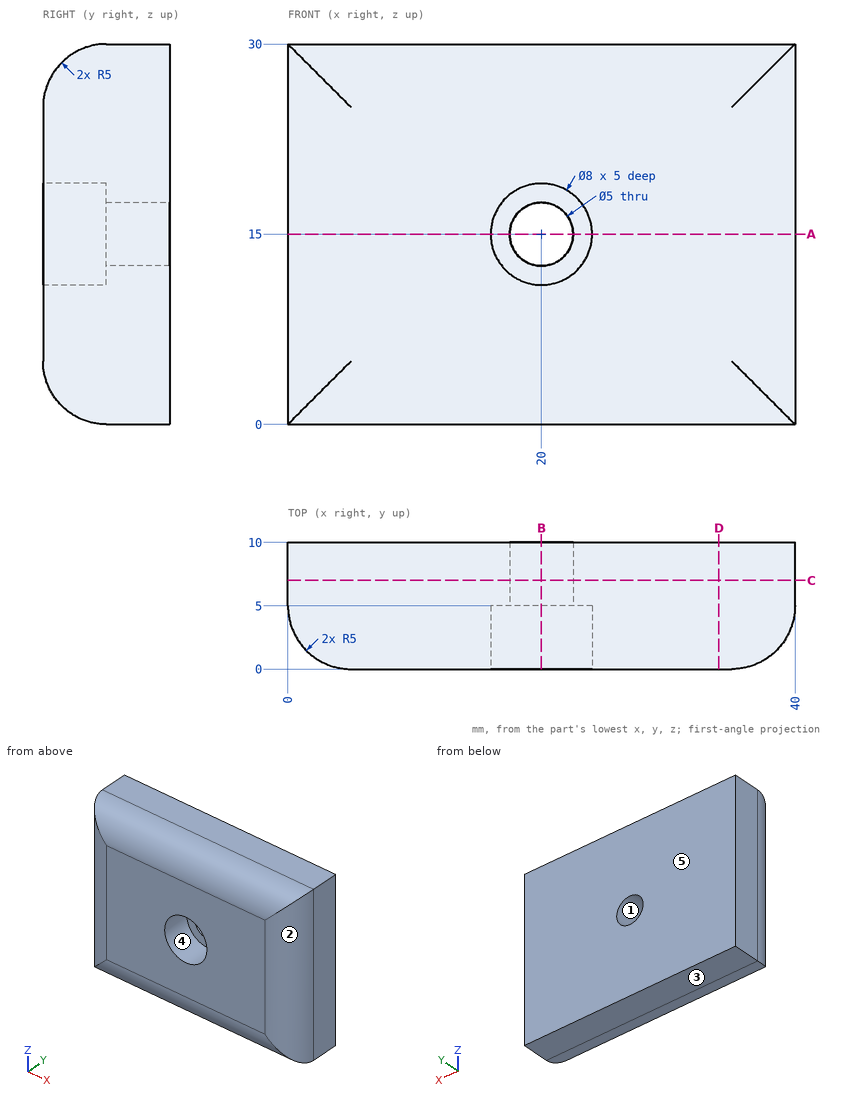
Geometry: see drawing. Coordinates: mm, zero at the bounding-box minimum. A direction names the side the tool comes from. Coordinates: 2 decimals unless noted, no trailing zeros. Loops run counter-clockwise (first coordinate to the right, second up) from the corner with the lowest first, then second, coordinate; pieces in that order, holes last. Notation, with made-up numbers: (-4.5, 7.25) -> (8.5, 7.25) arc R24 ccw to (8.5, 37.25) -> close; hole circle Ø5 at (31.5, -2.75). An arc over 180 degrees is marked (long way). Use a Markdown table: item, result.
1) Material intervals for line 1 along X through (y, z) = (7.5, 15); line 2 along X through (y, z) = (2.25, 15); line 3 along Z through (x, y) = (18.5, 6.5), sorted ascending. Write a range as from..to.
Results found:
| item | result |
|---|---|
| line 1 | x = 0..17.5, 22.5..40 |
| line 2 | x = 0.82..16, 24..39.18 |
| line 3 | z = 0..13, 17..30 |
2) Cut plane D-D (x = 34). Return the cut outline in (y, z).
Results found:
| item | result |
|---|---|
| outline | (0, 5) arc R5 ccw to (5, 0) -> (10, 0) -> (10, 30) -> (5, 30) arc R5 ccw to (0, 25) -> close |
3) Cut plane A-A (z = 15). Return the cut outline in (x, y), then the cut area to 3 significant figures.
Results found:
| item | result |
|---|---|
| outline | (0, 5) arc R5 ccw to (5, 0) -> (16, 0) -> (16, 5) -> (17.5, 5) -> (17.5, 10) -> (0, 10) -> close; (22.5, 5) -> (24, 5) -> (24, 0) -> (35, 0) arc R5 ccw to (40, 5) -> (40, 10) -> (22.5, 10) -> close |
| area | 324 mm2 |
4) Cut plane C-C (y = 7). Return the cut outline in (x, z), then the cut area to 3 significant figures.
Results found:
| item | result |
|---|---|
| outline | (0, 0) -> (40, 0) -> (40, 30) -> (0, 30) -> close; hole circle Ø5 at (20, 15) |
| area | 1,180 mm2 |
5) Cut plane B-B (x = 20). Return the cut outline in (y, z), then the cut area to 3 significant figures.
Results found:
| item | result |
|---|---|
| outline | (0, 5) arc R5 ccw to (5, 0) -> (10, 0) -> (10, 12.5) -> (5, 12.5) -> (5, 11) -> (0, 11) -> close; (0, 19) -> (5, 19) -> (5, 17.5) -> (10, 17.5) -> (10, 30) -> (5, 30) arc R5 ccw to (0, 25) -> close |
| area | 224 mm2 |
6) Pull-direction query (X, two-part tool) for the marked faces 1, 2 and 3; classes: released by +X, released by -X, zero draft, split by the parting line, or undercut.
Results found:
| item | result |
|---|---|
| face 1 | undercut |
| face 2 | released by +X |
| face 3 | zero draft |
7) Contact query for flat-ended pins moving along their axis: pin 1 (6 mm diameter, centred on y = 1.5, z = 22, fed in from +X); pin 2 (6 mm diameter, centred on x = 20, z = 15, fed in from -Y); pin 3 (9 mm diameter, centred on x = 21.5, z = 15.5, fed in from -Y). Output: stop coordinate, or through.
Results found:
| item | result |
|---|---|
| pin 1 | stops at x = 39.97 |
| pin 2 | stops at y = 5 |
| pin 3 | stops at y = 0 |
8) Access query for the marked faces 4 and 5. Directions: +Z, -Z, +X, -X, +Y, -Y. A direction counts if a zero-diameter tool reaches every point of the face in a straight line with its end or side. Return the directions, or none.
Results found:
| item | result |
|---|---|
| face 4 | -Y |
| face 5 | +Z, -Z, +X, -X, +Y |
